For this review, take the finished solid that the model builds, in its own axes (mm). A direction names the side the tool comes from. Give positions to 0.01 mm unless a question says otherwise; leave off trailing zeros. Loops run counter-clockwise (first coordinate to the right, second up) from the corner with the lowest first, then second, coordinate; pieces in that order, holes last. Notation, with made-up numbers: (73.25, 8.5) -> (128.25, 8.5) arc R28 cw to (128.25, 41.5) -> close; hole circle Ø11 at (-12.5, 36.25). An arc over 180 degrees is marked (long way). Answer as CSV lines item,"result". Start each with the question number.
Item 1: Machinability: for faces 1 (the face through (-26, 41, 3.175)), 2 (the face through (25.97, 29, 3.22)), which of the approach directions +Z, -Z, +X, -X, +Y, -Y give a long, thin tool a straight path to every point of the face, cutting with its end or side? Answer none if there is none.
Item 2: For L1, parallel to X at y = -19, z = 2.75; L2, parallel to Y at x = -14, z = 5.75; L3, parallel to Y at x = -12.7, z = 5.25, list the stretches that pass through material, from the lowest coordinate up. Write a range as from..to.
Item 3: Add section B-B on y = 0. State how many separate pieces and enclosed holes the cut face has, plus the area to 3 significant figures.
Item 4: The part is to be moulded in two halves that separate along Y. For faces 3 (the face through (28.58, 0.14, 3.22)), 4 (the face through (-34.92, 0.14, 3.22)), 5 (the face through (-6.445, 49.083, 1.565)), 6 (the face through (-1, 1, 6.35)), say which applies: +Y half, -Y half, draft (parallel to the pull), parting line (faces both ways), or undercut.
Item 5: Clearance check with flat-ended pins moving along their axes: P1, Ø7.5, axis at x = 31.75, y = 0, coming from the +Z side; P2, Ø1.5, axis at y = 15.5, z = 4, coming from the +X side; P3, Ø1, axis at y = -26, z = 3, coming from the -X side; P4, Ø2, axis at y = 19, z = 1.5, coming from the -X side. State where each tip first meets the part, or that it passes through.
Item 6: Add section C-C on x = 22.5. State the section outline as (y, z) points (3 decimals).
```python
from build123d import *

# Parameters (mm, degrees)
SKETCH1_R           = 49.5046
BOSS_EXTRUDE1_DEPTH = 3.175
SKETCH2_R           = 47.6885
BOSS_EXTRUDE2_DEPTH = 3.175
SKETCH3_R           = 6.35
SKETCH3_R_2         = 3.175
SKETCH3_R_3         = 4.7625
SKETCH3_R_4         = 2.54
CUT_EXTRUDE1_DEPTH  = 71.297463271


with BuildPart() as part:
    # Sketch1 → Boss-Extrude1 (new body)
    with BuildSketch(Plane.XY):
        Circle(SKETCH1_R)
    extrude(amount=BOSS_EXTRUDE1_DEPTH)

    # Sketch2 → Boss-Extrude2 (add)
    with BuildSketch(Plane.XY.offset(3.175)):
        Circle(SKETCH2_R)
    extrude(amount=BOSS_EXTRUDE2_DEPTH)

    # Sketch3 → Cut-Extrude1 (cut, through all)
    with BuildSketch(Plane.XY.offset(6.35)):
        with Locations((-12.7, -31.235352443)):
            Circle(SKETCH3_R)
        with Locations((12.7, -31.235352443)):
            Circle(SKETCH3_R)
        with Locations((-31.75, 0)):
            Circle(SKETCH3_R_2)
        with Locations((31.75, 0)):
            Circle(SKETCH3_R_2)
        with Locations((0, 6.35)):
            Circle(SKETCH3_R_3)
        with Locations((-14.850390051, -11.029456704)):
            Circle(SKETCH3_R_2)
        with Locations((-23.622, 29.972)):
            Circle(SKETCH3_R_4)
        with Locations((23.622, 29.972)):
            Circle(SKETCH3_R_4)
        with Locations((23.622, -17.272)):
            Circle(SKETCH3_R_4)
        with Locations((-23.622, -17.272)):
            Circle(SKETCH3_R_4)
    extrude(amount=-CUT_EXTRUDE1_DEPTH, mode=Mode.SUBTRACT)


solid = part.part
```
Computed values:
1,face 1,"+Z"
1,face 2,"+Z, -Z"
2,L1,"-45.71..-25.48, -21.76..21.76, 25.48..45.71"
2,L2,"-45.59..-37.45, -25.02..-14.09, -7.97..45.59"
2,L3,"-45.97..-37.59, -24.89..-13.37, -8.69..45.97"
3,separate pieces,"3"
3,enclosed holes,"0"
3,area,"537 mm²"
4,face 3,"undercut"
4,face 4,"undercut"
4,face 5,"parting line"
4,face 6,"draft"
5,P1,"z = 6.35"
5,P2,"x = 45.35"
5,P3,"x = -42.43"
5,P4,"x = -46.12"
6,outline,"(-44.096, 0) -> (-19.551, 0) -> (-19.551, 6.35) -> (-42.047, 6.35) -> (-42.047, 3.175) -> (-44.096, 3.175) -> close; (-14.993, 0) -> (27.693, 0) -> (27.693, 6.35) -> (-14.993, 6.35) -> close; (32.251, 0) -> (44.096, 0) -> (44.096, 3.175) -> (42.047, 3.175) -> (42.047, 6.35) -> (32.251, 6.35) -> close"
